Work out the finished part from the listing and answer in its coordinate system (mm). A direction names the side the tool comes from. Coordinates: 2 decimals unless noted, no trailing zeros. Write each loop counter-clockwise with the first axis right and the second up, starting at its lowest first coordinate (ties: lowest second). Pieces come first, ordered by that corner, then holes. Notation, with made-up numbers: (54, 5) - (67, 5) arc R11 ccw to (67, 13) - close; hole circle Ø3 at (-38, 4). An arc over 180 degrees is marked (long way). Use a Markdown table: item, result. Add a question column.
(1) The part is cut by section B-B, the plane y = -153. Give the vertices of the cut face in (x, z) (3 decimals), then the cut area to 3 significant figures.
(2) The part is cut by section A-A, the plane z = 1.15. Give the vertices of the cut face in (x, y) (3 decimals).
(3) A tool of negligible diameter and unlimited length cuts with its end or side. For faces 5 (the face through (-144, -161, 0.145)), 6 (the face through (-144, 3, -0.145)), 7 (the face through (-135.852, 142.138, -1.131)), from which of +Z, -Z, +X, -X, +Y, -Y can it reach the whole face along a straight path? Write none if from no direction.
(4) Find the intervals of material crossed by line 1 (Z direction, x = -142, y = 18) (3 decimals); line 2 (Y direction, x = -144.25, z = 1.4) (3 decimals); line 3 (Y direction, x = -147, z = -1.75), in increasing order. Write a range as from..to.
(5) For a pull along Y with two mould halves and no side action, classify faces 1 (the face through (-152.148, 142.138, -1.131)), 2 (the face through (-143.23, 129.3, -1.16)), 3 (the face through (-136.007, -173.003, 1.131)), 4 (the face through (-144, -161, 2.145)) as released by +Y, released by -Y, zero draft, split by the parting line, or undercut.
(6) Given pin 1 Ø4 at (x, y) = (-152, -49.5) entering from +Z (3 decimals); pin 2 Ø6.5 at (x, y) = (-148, -155) entering from -Z (3 decimals); pin 3 Ø1.5 at (x, z) = (-147, 0.5) entering from +Y, each flat-ended and moving along its own axis, determine where each tip first touches the part or whether it passes through.
from build123d import *

# Parameters (mm, degrees)
BASE_FLANGE1_DEPTH      = 11
FILLET1_R               = 10
CUT_EXTRUDE1_DEPTH      = 290.218332925
CUT_EXTRUDE1_DEPTH_BACK = 290.218332925
SKETCH7_R               = 5.894184215
SKETCH7_R_2             = 1
BODY_MOVE_COPY1_ANGLE   = 120


# Sheet-metal steps are written as plain solids
with BuildPart() as part:
    # Sketch2 → Base-Flange1 (new, symmetric)
    with BuildSketch(Plane.XY):
        with BuildLine():
            Line((-289, 0), (-0.1, 0))
            ThreePointArc((-0.1, 0), (-0.029289322, 0.029289322), (0, 0.1))
            Line((0, 0.1), (0, 0.19))
            ThreePointArc((0, 0.19), (0.61507576, 1.67492424), (2.1, 2.29))
            Line((2.1, 2.29), (32, 2.29))
            Line((32, 2.29), (32, 0.29))
            Line((32, 0.29), (2.1, 0.29))
            ThreePointArc((2.1, 0.29), (2.029289322, 0.260710678), (2, 0.19))
            Line((2, 0.19), (2, 0.1))
            ThreePointArc((2, 0.1), (1.38492424, -1.38492424), (-0.1, -2))
            Line((-0.1, -2), (-289, -2))
            Line((-289, -2), (-289, 0))
        make_face()
    extrude(amount=BASE_FLANGE1_DEPTH, both=True)

    # Fillet1
    fillet1_edges = [part.edges().sort_by_distance(p)[0] for p in [
        (-289, -1, -11),
        (32, 1.29, -11),
        (-289, -1, 11),
        (32, 1.29, 11),
    ]]
    fillet(fillet1_edges, radius=FILLET1_R)

    # Sketch7 → Cut-Extrude1 (cut, two sides: drawn at the far end of the back side and taken through both)
    with BuildSketch(Plane(origin=(0, 0, 0), x_dir=(1, 0, 0), z_dir=(0, 1, 0)).offset(-CUT_EXTRUDE1_DEPTH_BACK)):
        with Locations(Location((-279, 0, 0), (0, 0, 270))):
            Circle(SKETCH7_R)
        with Locations(Location((21.883026743, 0.116566496, 0), (0, 0, 270))):
            Circle(SKETCH7_R_2)
    extrude(amount=CUT_EXTRUDE1_DEPTH + CUT_EXTRUDE1_DEPTH_BACK, mode=Mode.SUBTRACT)


with BuildPart() as part_1:
    # Body-Move/Copy1: moved
    add(part.part.moved(Location((0, 0, 0))).rotate(Axis((-95.951666667, -47.903333333, -48.048333333), (0.5773502691899637, -0.5773502691896031, -0.5773502691893106)), BODY_MOVE_COPY1_ANGLE))


solid = part_1.part
Model answer:
| question | item | result |
|---|---|---|
| 1 | outline | (-155, 0.145) - (-133, 0.145) - (-133, 2.145) - (-155, 2.145) - close |
| 1 | area | 44.0 mm^2 |
| 2 | outline | (-155, -165.855) arc R10 ccw to (-145, -175.855) - (-143, -175.855) arc R10 ccw to (-133, -165.855) - (-133, -144.169) - (-155, -144.169) - close; hole circle Ø2 at (-143.883, -165.738) |
| 3 | face 5 | -Z, +X, -X, -Y |
| 3 | face 6 | +Z, +X, -X, +Y |
| 3 | face 7 | +Z, -Z, +X, +Y |
| 4 | line 1 | -2.145..-0.145 |
| 4 | line 2 | -175.855..-166.668, -164.808..-144.351 |
| 4 | line 3 | -144.98..130.07, 140.22..144.94 |
| 5 | face 1 | released by +Y |
| 5 | face 2 | undercut |
| 5 | face 3 | released by -Y |
| 5 | face 4 | zero draft |
| 6 | pin 1 | z = -0.145 |
| 6 | pin 2 | z = 0.145 |
| 6 | pin 3 | y = 145.01 |
